For this review, take the finished solid that the model builds, in its own axes (mm). Give positions to 0.01 mm unless a question says otherwise; leave off trailing zeros. Write each loop counter-clockwise with the first axis right and the second up, starting at its lowest first coordinate (ties: lowest second). Pieces come first, ordered by that corner, then holes.
1) Wall thickness on line 1 along X through (y, z) = (-1492.5, 80); line 2 along Y through (x, z) = (-640, 46.5); line 3 along Y through (x, z) = (-474, 28): over which ranges is each line inside the solid? List them lowest first.
2) We need section D-D on y = -1098. Give the boundary of the cut face in (x, z), and give its area (4 significant figures).
3) We need section B-B on z = 106. Give the boundary of the cut face in (x, y), and give its area (4 significant figures).
4) We need section A-A on y = -1424.5. Give the boundary of the cut face in (x, z).
5) We need section C-C on x = -499. Give the boundary of the cut face in (y, z).
6) For P1, Ø1.5, axis at x = -154.5, z = 109.5, coming from the -Y side; P2, Ø6, axis at x = -287.5, z = 23.5, coming from the +Y side; P3, Ø1.5, axis at x = -721, y = -1572, coming from the -Z side; P4, Ø12, axis at x = -355, z = 13.5, coming from the -Y side, all flat-tipped, find the tip position at first contact; note any pin that passes through.
from build123d import *

# Parameters (mm, degrees)
BOSS_EXTRUDE1_DEPTH = 150
SKETCH4_W           = 690
SKETCH4_H           = 1970
CUT_EXTRUDE1_DEPTH  = 40
SKETCH5_W           = 30
SKETCH5_H           = 170
CUT_EXTRUDE2_DEPTH  = 5
CUT_EXTRUDE3_DEPTH  = 3


with BuildPart() as part:
    # Sketch1 → Boss-Extrude1 (new body)
    with BuildSketch(Plane.XY):
        Polygon((0, 0), (-750, 0), (-750, -2000), (-700, -2000), (-700, -50), (-50, -50), (-50, -2000), (0, -2000), align=None)
    extrude(amount=BOSS_EXTRUDE1_DEPTH)

    # Sketch4 → Cut-Extrude1 (cut)
    with BuildSketch(Plane(origin=(0, 0, 0), x_dir=(-1, 0, 0), z_dir=(0, 0, -1))):
        with Locations((375, -1015)):
            Rectangle(SKETCH4_W, SKETCH4_H)
    extrude(amount=-CUT_EXTRUDE1_DEPTH, mode=Mode.SUBTRACT)

    # Sketch5 → Cut-Extrude2 (cut)
    with BuildSketch(Plane.ZY.offset(30)):
        with Locations((20, -1045)):
            Rectangle(SKETCH5_W, SKETCH5_H)
    extrude(amount=-CUT_EXTRUDE2_DEPTH, mode=Mode.SUBTRACT)

    # Sketch6 → Cut-Extrude3 (cut)
    with BuildSketch(Plane(origin=(-720, 0, 0), x_dir=(0, 0, -1), z_dir=(1, 0, 0))):
        with BuildLine():
            Line((-35, -120), (-35, -210))
            Line((-35, -210), (0, -210))
            Line((0, -210), (0, -160))
            Line((0, -160), (-5, -160))
            Line((-5, -160), (-5, -120))
            ThreePointArc((-5, -120), (-20, -110), (-35, -120))
        make_face()
        with BuildLine():
            Line((-35, -1510), (-35, -1600))
            Line((-35, -1600), (0, -1600))
            Line((0, -1600), (0, -1550))
            Line((0, -1550), (-5, -1550))
            Line((-5, -1550), (-5, -1510))
            ThreePointArc((-5, -1510), (-20, -1500), (-35, -1510))
        make_face()
    extrude(amount=-CUT_EXTRUDE3_DEPTH, mode=Mode.SUBTRACT)


solid = part.part
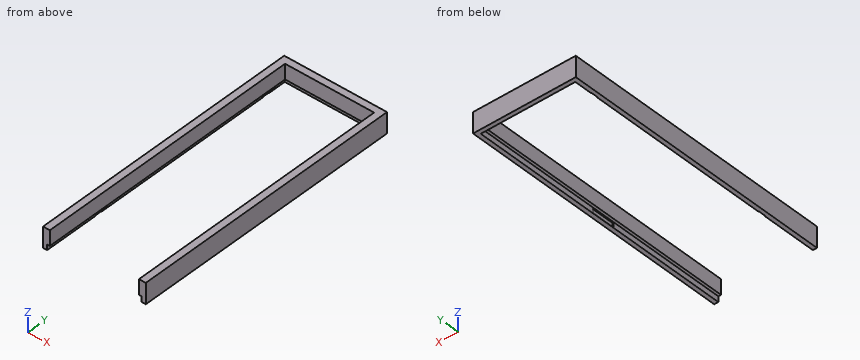
Results list:
1. line 1: x = -750 to -700, -50 to 0
1. line 2: y = -50 to 0
1. line 3: y = -30 to 0
2. outline: (-750, 0) - (-720, 0) - (-720, 40) - (-700, 40) - (-700, 150) - (-750, 150) - close; (-50, 40) - (-30, 40) - (-30, 35) - (-25, 35) - (-25, 5) - (-30, 5) - (-30, 0) - (0, 0) - (0, 150) - (-50, 150) - close
2. area: 13,250 mm2
3. outline: (-750, -2000) - (-700, -2000) - (-700, -50) - (-50, -50) - (-50, -2000) - (0, -2000) - (0, 0) - (-750, 0) - close
3. area: 232,500 mm2
4. outline: (-750, 0) - (-720, 0) - (-720, 40) - (-700, 40) - (-700, 150) - (-750, 150) - close; (-50, 40) - (-30, 40) - (-30, 0) - (0, 0) - (0, 150) - (-50, 150) - close
5. outline: (-50, 40) - (-30, 40) - (-30, 0) - (0, 0) - (0, 150) - (-50, 150) - close
6. P1: stops at y = -50
6. P2: stops at y = 0
6. P3: stops at z = 35
6. P4: stops at y = -30
